from build123d import *

# Parameters (mm, degrees)
SKETCH1_R           = 2.1
BOSS_EXTRUDE1_DEPTH = 4
FILLET1_R           = 0.2


with BuildPart() as part:
    # Sketch1 → Boss-Extrude1 (new body)
    with BuildSketch(Plane.XY):
        Polygon((4.618802154, 0), (2.309401077, 4), (-2.309401077, 4), (-4.618802154, 0), (-2.309401077, -4), (2.309401077, -4), align=None)
        Circle(SKETCH1_R, mode=Mode.SUBTRACT)
    extrude(amount=BOSS_EXTRUDE1_DEPTH)

    # Fillet1
    fillet1_edges = [part.edges().sort_by_distance(p)[0] for p in [
        (0, 4, 4),
        (-3.464101615, 2, 4),
        (-3.464101615, -2, 4),
        (-2.1, 0, 0),
        (-2.1, 0, 4),
        (0, -4, 4),
        (3.464101615, -2, 4),
        (0, -4, 0),
        (-3.464101615, -2, 0),
        (-3.464101615, 2, 0),
        (3.464101615, 2, 4),
        (0, 4, 0),
        (3.464101615, 2, 0),
        (3.464101615, -2, 0),
    ]]
    fillet(fillet1_edges, radius=FILLET1_R)


solid = part.part
Model file for the job. Use its own axes, mm. Round coordinates to 2 decimals unless told otherwise and drop trailing zeros. Order: outer loops, then holes, each group sorted by start corner. A loop starts at its lowest first (then second) coordinate and runs counter-clockwise, first axis right, second up.
(1) Drill centre lines: line 1 (Y direction, x = 0, z = 1.9); line 2 (Y direction, x = -2.75, z = 1.9); line 3 (Y direction, x = 0.5, z = 0.2). Where is each one in solid material? Low to high.
(2) Band-saw the part on A-A (z = 2.1). List the corners of the cut face in (x, y), then the cut area to 3 significant figures.
(3) Pull direction X, two halves, no side cores. Call faces 1 (the face through (2, 2, 4)), 2 (the face through (3.43, -1.94, 3.94)), 3 (the face through (2.003, 0.631, 1.975)), 4 (the face through (-3.48, -1.97, 1.97)): released by +X, released by -X, zero draft, split by the parting line, or undercut.
(4) Pin check, flat tips, straight feed: pin 1 (1.5 mm diameter, centred on x = 1.5, y = 0, fed in from +Z); pin 2 (1.5 mm diameter, centred on x = -1, y = 0.5, fed in from -Z). Stop position of each tip, or through.
(5) Band-saw the part on B-B (x = 0). List the corners of the cut face in (y, z).
Verdict:
1. line 1: y = -4 to -2.1, 2.1 to 4
1. line 2: y = -3.24 to 3.24
1. line 3: y = -4 to -2.04, 2.04 to 4
2. outline: (-4.62, 0) - (-2.31, -4) - (2.31, -4) - (4.62, 0) - (2.31, 4) - (-2.31, 4) - close; hole circle Ø4.2 at (0, 0)
2. area: 41.6 mm2
3. face 1: zero draft
3. face 2: released by +X
3. face 3: undercut
3. face 4: released by -X
4. pin 1: stops at z = 3.99
4. pin 2: passes through
5. outline: (-4, 0.2) arc R0.2 ccw to (-3.8, 0) - (-2.3, 0) arc R0.2 ccw to (-2.1, 0.2) - (-2.1, 3.8) arc R0.2 ccw to (-2.3, 4) - (-3.8, 4) arc R0.2 ccw to (-4, 3.8) - close; (2.1, 0.2) arc R0.2 ccw to (2.3, 0) - (3.8, 0) arc R0.2 ccw to (4, 0.2) - (4, 3.8) arc R0.2 ccw to (3.8, 4) - (2.3, 4) arc R0.2 ccw to (2.1, 3.8) - close
